Answer from the drawing. Dimensions are ordinates in mm from the lowest x, y and z of the part. Give positions to 0.01 mm unless a question says otherwise; leave off trailing zeros. Write each loop counter-clockwise with the first axis right and the second up, starting at its lowest first coordinate (ties: lowest second). Pieces come first, ordered by that corner, then holes.
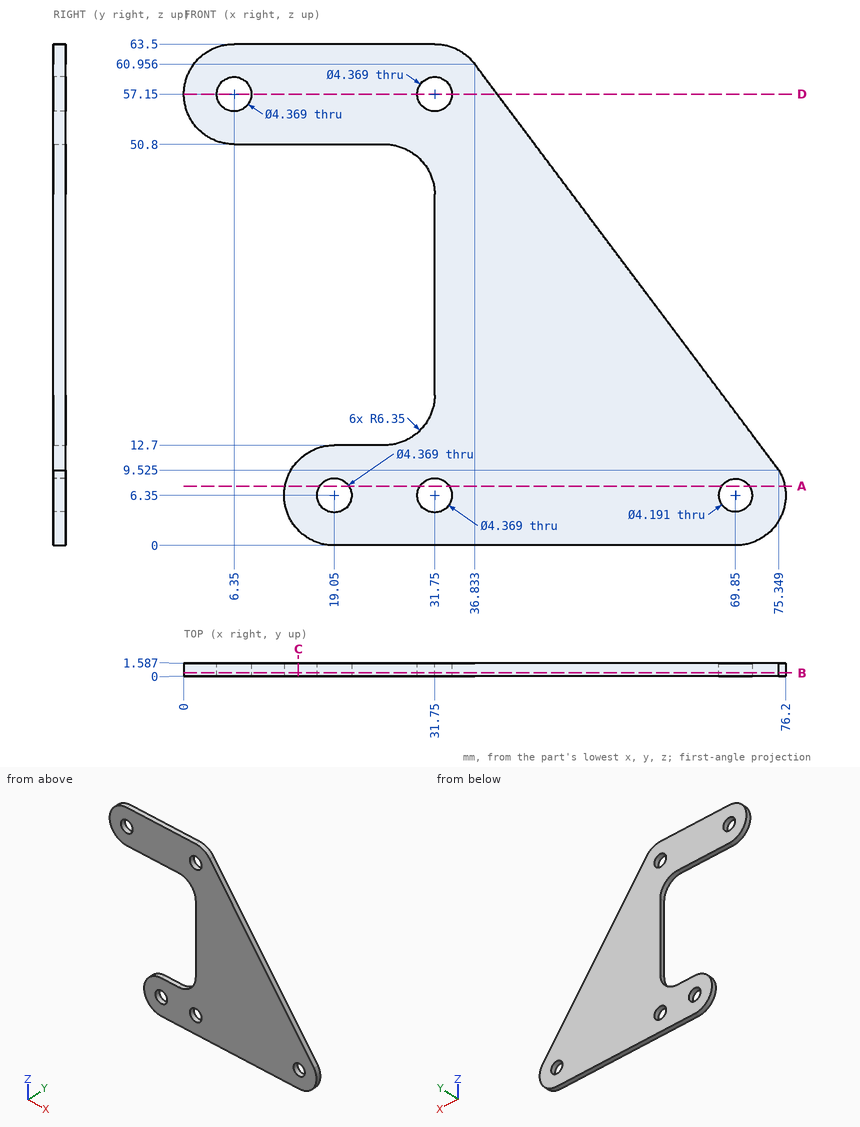
Item 1: Section A-A (z = 7.5) is taken. Write down the section's boundary in (x, y) (1 decimal).
Result set:
outline: (12.8, 0) - (17.2, 0) - (17.2, 1.6) - (12.8, 1.6) - close; (20.9, 0) - (29.9, 0) - (29.9, 1.6) - (20.9, 1.6) - close; (33.6, 0) - (68.1, 0) - (68.1, 1.6) - (33.6, 1.6) - close; (71.6, 0) - (76.1, 0) - (76.1, 1.6) - (71.6, 1.6) - close
Item 2: Each of these flat-tipped pins is pushed along its axis until it touches: pin 1 Ø5 at (x, z) = (6.35, 57.15) entering from -Y; pin 2 Ø4 at (x, z) = (69.85, 6.35) entering from +Y. Where does it stop, or does it pass through?
Result set:
pin 1: stops at y = 0
pin 2: passes through
Item 3: Section B-B (y = 0.4) is taken. Give the number of separate pieces and of enclosed holes in the cut face, and give its area (3 significant figures).
Result set:
separate pieces: 1
enclosed holes: 5
area: 2,230 mm2
Item 4: Section D-D (z = 57.15) is taken. Write down the section's boundary in (x, y) (1 decimal).
Result set:
outline: (0, 0) - (4.2, 0) - (4.2, 1.6) - (0, 1.6) - close; (8.5, 0) - (29.6, 0) - (29.6, 1.6) - (8.5, 1.6) - close; (33.9, 0) - (39.7, 0) - (39.7, 1.6) - (33.9, 1.6) - close
Item 5: Section C-C (x = 14.5) is taken. Write down the section's boundary in (y, z).
Result set:
outline: (0, 1.92) - (1.59, 1.92) - (1.59, 10.78) - (0, 10.78) - close; (0, 50.8) - (1.59, 50.8) - (1.59, 63.5) - (0, 63.5) - close
Item 6: Find the intervals of material crossed by line 1 along X through (y, z) = (0.95, 6.5); line 2 along Z through (x, y) = (18, 0.55) (1 decimal); line 3 along Z through (x, y) = (69.85, 1.1) (1 decimal), in increasing order.
Result set:
line 1: x = 12.7 to 16.87, 21.23 to 29.57, 33.93 to 67.76, 71.94 to 76.2
line 2: z = 0.1 to 4.4, 8.3 to 12.6, 50.8 to 63.5
line 3: z = 0 to 4.3, 8.4 to 16.9
